from build123d import *

# Parameters (mm, degrees)
SKETCH_2_W          = 63
SKETCH_2_H          = 43
SKETCH_2_R          = 1.75
SKETCH_2_R_2        = 12.5
SKETCH_2_R_3        = 2.75
EXTRUDE_1_DEPTH     = 5
SKETCH_3_W          = 63
SKETCH_3_H          = 5
EXTRUDE_2_DEPTH     = 25
SKETCH_4_R          = 4.25
CUT_EXTRUDE_2_DEPTH = 25
SKETCH_5_R          = 7.75
SKETCH_5_R_2        = 4.25
EXTRUDE_3_DEPTH     = 10
EXTRUDE_4_DEPTH     = 5
EXTRUDE_5_DEPTH     = 5
SKETCH_10_R         = 2.75
CUT_EXTRUDE_3_DEPTH = 75.939521233
SKETCH_11_W         = 20
SKETCH_11_H         = 5
EXTRUDE_6_DEPTH     = 5
CHAMFER_1_SIZE      = 3


with BuildPart() as part:
    # 草图2 → 凸台-拉伸1 (new body)
    with BuildSketch(Plane.XY):
        with Locations((11.527972028, -9.531468531)):
            Rectangle(SKETCH_2_W, SKETCH_2_H)
        with Locations((-13.972027972, 5.968531469)):
            Circle(SKETCH_2_R, mode=Mode.SUBTRACT)
        with Locations((17.027972028, 5.968531469)):
            Circle(SKETCH_2_R, mode=Mode.SUBTRACT)
        with Locations((17.027972028, -25.031468531)):
            Circle(SKETCH_2_R, mode=Mode.SUBTRACT)
        with Locations((-13.972027972, -25.031468531)):
            Circle(SKETCH_2_R, mode=Mode.SUBTRACT)
        with Locations((1.527972028, -9.531468531)):
            Circle(SKETCH_2_R_2, mode=Mode.SUBTRACT)
        with Locations((33.027972028, 1.968531469)):
            Circle(SKETCH_2_R_3, mode=Mode.SUBTRACT)
        with Locations((33.027972028, -21.031468531)):
            Circle(SKETCH_2_R_3, mode=Mode.SUBTRACT)
    extrude(amount=EXTRUDE_1_DEPTH)

    # 草图3 → 凸台-拉伸2 (add)
    with BuildSketch(Plane.XZ.offset(31.031468531)):
        with Locations((11.527972028, 2.5)):
            Rectangle(SKETCH_3_W, SKETCH_3_H)
    extrude(amount=EXTRUDE_2_DEPTH)

    # 草图4 → 切除-拉伸2 (cut)
    with BuildSketch(Plane.XY.offset(5)):
        with Locations((1.527972028, -48.031468531)):
            Circle(SKETCH_4_R)
    extrude(amount=-CUT_EXTRUDE_2_DEPTH, mode=Mode.SUBTRACT)

    # 草图5 → 凸台-拉伸3 (add)
    with BuildSketch(Plane(origin=(0, 0, 0), x_dir=(-1, 0, 0), z_dir=(0, 0, -1))):
        with Locations(Location((-1.527972028, -48.031468531, 0), (0, 0, 180))):
            Circle(SKETCH_5_R)
        with Locations(Location((-1.527972028, -48.031468531, 0), (0, 0, 180))):
            Circle(SKETCH_5_R_2, mode=Mode.SUBTRACT)
    extrude(amount=EXTRUDE_3_DEPTH)

    # 草图7 → 凸台-拉伸4 (add)
    with BuildSketch(Plane(origin=(0, 11.968531469, 0), x_dir=(1, 0, 0), z_dir=(0, 1, 0))):
        Polygon((-19.972027972, -5), (-19.472027972, 5), (23.027972028, 20), (23.027972028, -5), align=None)
    extrude(amount=EXTRUDE_4_DEPTH)

    # 草图8 → 凸台-拉伸5 (add)
    with BuildSketch(Plane(origin=(0, -31.031468531, 0), x_dir=(-1, 0, 0), z_dir=(0, -1, 0))):
        Polygon((-23.027972028, 20), (-23.027972028, 0), (19.722027972, 0), (19.472027972, 5), align=None)
    extrude(amount=EXTRUDE_5_DEPTH)

    # 草图10 → 切除-拉伸3 (cut, through all)
    with BuildSketch(Plane.XY.offset(5)):
        with Locations((33.027972028, -44.031468531)):
            Circle(SKETCH_10_R)
    extrude(amount=-CUT_EXTRUDE_3_DEPTH, mode=Mode.SUBTRACT)

    # 草图11 → 凸台-拉伸6 (add)
    with BuildSketch(Plane(origin=(0, 11.968531469, 0), x_dir=(1, 0, 0), z_dir=(0, 1, 0))):
        with Locations((33.027972028, -2.5)):
            Rectangle(SKETCH_11_W, SKETCH_11_H)
    extrude(amount=EXTRUDE_6_DEPTH)

    # 倒角1
    chamfer_1_edges = [part.edges().sort_by_distance(p)[0] for p in [
        (-19.972027972, -56.031468531, 2.5),
        (-19.722027972, 16.968531469, 0),
    ]]
    chamfer(chamfer_1_edges, length=CHAMFER_1_SIZE)


solid = part.part
Read the model definition and answer for the solid it produces. Units are mm, in the model's axes. A direction names the side the tool comes from. Coordinates: 2 decimals unless noted, no trailing zeros. Write each loop counter-clockwise with the first axis right and the second up, starting at its lowest first coordinate (ties: lowest second). Pieces come first, ordered by that corner, then holes. Notation, with made-up numbers: (33, 18.5) -> (84, 18.5) arc R20 ccw to (84, 36.5) -> close; hole circle Ø4 at (-29, -12). An arc over 180 degrees is marked (long way). Return JSON: item names as keys, results as strings.
(1) The part is cut by section A-A on y = -4.5. Give the vertices of the cut face in (x, z), then the cut area to 3 significant figures.
Answers below:
{"outline": "(-19.97, 0) -> (-9.91, 0) -> (-9.91, 5) -> (-19.97, 5) -> close; (12.97, 0) -> (43.03, 0) -> (43.03, 5) -> (12.97, 5) -> close", "area": "201 mm^2"}
(2) For a pull along Y with two mould halves and no side action, classify faces 1 (the flat face through (11, -20, 5)), 2 (the flat face through (13, -56.031, 3)), 3 (the cylindrical face through (-1.182, -21.734, 2.465)), 4 (the cylindrical face through (31.001, -19.173, 2.465)) as pulls with the +Y half, pulls with the -Y half, needs draft (parallel to the pull), parting line crosses it, or undercut.
Answers below:
{"face 1": "needs draft", "face 2": "pulls with the -Y half", "face 3": "undercut", "face 4": "undercut"}
(3) The part is cut by section B-B on z = 1.5. State how many separate pieces and enclosed holes the cut face has, then the cut area to 3 significant figures.
Answers below:
{"separate pieces": "1", "enclosed holes": "9", "area": "3,930 mm^2"}
(4) The part is cut by section D-D on z = -15.75. Give the vertices of the cut face in (x, y), then the cut area to 3 significant figures.
Answers below:
{"outline": "(10.99, -36.03) -> (23.03, -36.03) -> (23.03, -31.03) -> (10.99, -31.03) -> close; (10.99, 11.97) -> (23.03, 11.97) -> (23.03, 16.97) -> (10.99, 16.97) -> close", "area": "120 mm^2"}
(5) Each of these flat-tipped pins is pushed along its axis until it touches: P1, Ø19, axis at x = 4, y = -16, coming from the -Z side; P2, Ø1, axis at x = 12.5, z = -17, coming from the +Y side; P3, Ø3, axis at x = -13, z = -8.5, coming from the +Y side; P4, Ø4, axis at y = -33, z = -14.5, coming from the +X side. Where does it stop, or does it pass through?
Answers below:
{"P1": "z = 0", "P2": "through", "P3": "y = 16.97", "P4": "x = 23.03"}
(6) Consider line 1 along Y through (x, z) = (35.5, 3.25); line 2 along Y through (x, z) = (-3, -1); line 3 along Y through (x, z) = (19, -8.25). Determine where each line is inside the solid, lowest interval first. Write a range as from..to.
Answers below:
{"line 1": "-56.03..-45.24, -42.83..-22.24, -19.83..0.76, 3.17..16.97", "line 2": "-54.32..-41.74, -36.03..-31.03, 11.97..16.97", "line 3": "-36.03..-31.03, 11.97..16.97"}
(7) Which of the six approach directions +Z, -Z, +X, -X, +Y, -Y give full straight-line access (tool end or side, diameter ignored) to faces 5 (the flat face through (-19.726, 12.955, 0.07)), 6 (the flat face through (-19.972, -20, 2)), 7 (the flat face through (7, 11.969, -8)), 8 (the flat face through (23.028, -33, -10))?
Answers below:
{"face 5": "-Z, -X, +Y", "face 6": "+Z, -Z, -X, +Y, -Y", "face 7": "-Z, +X, -X", "face 8": "-Z, +X, +Y, -Y"}
(8) The part is cut by section C-C on x = -8.5. Give the vertices of the cut face in (y, z).
Answers below:
{"outline": "(-56.03, 0) -> (-36.03, 0) -> (-36.03, -8.87) -> (-31.03, -8.87) -> (-31.03, 0) -> (-16.99, 0) -> (-16.99, 5) -> (-56.03, 5) -> close; (-2.07, 0) -> (11.97, 0) -> (11.97, -8.87) -> (16.97, -8.87) -> (16.97, 5) -> (-2.07, 5) -> close"}
